Design review of the part built by this model. Coordinates are the model's own, in mm. A direction names the side the tool comes from. Give positions to 0.01 mm unless a question says otherwise; leave off trailing zeros. Loops run counter-clockwise (first coordinate to the right, second up) from the corner with the lowest first, then second, coordinate; pieces in that order, holes last. Notation, with made-up numbers: (72.25, 57.25) - (94.25, 57.25) arc R12 cw to (94.25, 67.25) - close; hole circle Ø6 at (-27, -7.75). An arc over 180 degrees is marked (long way). Write each question's results on one line, items separated by ' | '.
Autodesk Inventor part; units mm, degrees
ref_plane "Work Plane1" through (0, -13.8, 0) normal (1, 0, 0) x (0, 0, 1)
ref_plane "YZ Plane" through (0, 0, 0) normal (1, 0, 0) x (0, 1, 0)
ref_plane "XZ Plane" through (0, 0, 0) normal (0, 1, 0) x (-1, 0, 0)
sketch "Sketch1" plane through (0, 0, 0) normal (0, 0, 1) x (1, 0, 0)
  arc A0 (9.4421, -21.6827) -> (-9.4421, -21.6827) centre (0, -13.8) ccw
  line L0 (0, 15.1128) -> (0, -73.1766)
  line L1 (-45.5, 0) -> (45.5, 0)
  line L2 (-4.9645, 1.7) -> (1.5024, 1.7) construction
  arc A1 (4.998, -26.8243) -> (-4.998, -26.8243) centre (0, -13) ccw
  line L3 (0, -1.5) -> (-5.3069, -1.5) construction
  line L4 (0, -13) -> (-6.8324, -26.0157) construction
  line L5 (-6.8324, -26.0157) -> (-20.0146, -19.0959) construction
  line L6 (-5.6007, -23.6693) -> (-15.85, -18.2891) construction
  circle A2 centre (-5.6007, -23.6693) radius 1
  arc A3 (-3.8298, -24.5989) -> (-6.7537, -22.0352) centre (-5.6007, -23.6693) ccw
  arc A4 (-9.4421, -21.6827) -> (-6.7537, -22.0352) centre (-7.9068, -20.401) ccw
  line L7 (-3.8298, -24.5989) -> (-4.998, -26.8243)
  circle A5 centre (5.6007, -23.6693) radius 1
  arc A6 (6.7537, -22.0352) -> (3.8298, -24.5989) centre (5.6007, -23.6693) ccw
  arc A7 (6.7537, -22.0352) -> (9.4421, -21.6827) centre (7.9068, -20.401) ccw
  line L8 (3.8298, -24.5989) -> (4.998, -26.8243)
  point P0 (-12.9705, -19.8007)
  point P1 (6.8324, -26.0157)
  dimension "d8" = 0.8
  dimension "d38" = 3.2
  dimension "d39" = 13
  dimension "d43" = 14.7
  dimension "d45" = 2.65
  dimension "d46" = 2
  dimension "d47" = 4.998
  dimension "d48" = 2
  dimension "d49" = 2
extrude "Body" add sketch "Sketch1" along normal blind 1.5
ref_plane "Work Plane1" through (0, -13.8, 0) normal (1, 0, 0) x (0, 0, 1)
equation "\"d8\" = 0.25 * SRB1"
equation "\"d38\" = SRB1"
equation "\"d39\" = 0.5 * WD"
equation "\"d43\" = 0.5 * ND"
equation "\"d45\" = 0.5 * SRB2"
equation "\"d46\" = SD5"
equation "\"d47\" = 0.17 * ND"
equation "\"d48\" = SD5"
equation "\"d49\" = SD5"
equation "\"d2\" = SD"
equation "\"WD\" = WDMIN"
equation "\"SD\" = 1.5"
equation "\"SRB1\" = 3.2"
equation "\"ND\" = 29.4"
equation "\"SRB2\" = 5.3"
equation "\"SD5\" = 2"
equation "\"WDMIN\" = 26"
equation "\"SD6\" = 30.1"
equation "\"NND\" = 28"
equation "\"WDMAX\" = NND"
properties part number "DIN 472 - 28 x 1.5" material "Steel, Mild"
(1) Take a section at D-D on x = 0. Give the boundary of the cut face in (y, z), plus the area to 3 significant figures.
Answers below:
outline: (-1.5, 0) - (1.7, 0) - (1.7, 1.5) - (-1.5, 1.5) - close | area: 4.80 mm2
(2) Take a section at B-B on z = 0.25. Give the boundary of the cut face in (x, y), plus the area to 3 significant figures.
Answers below:
outline: (-9.44, -21.68) arc R12.3 cw (long way) to (9.44, -21.68) arc R2 cw to (6.75, -22.04) arc R2 ccw to (3.83, -24.6) - (5, -26.82) arc R14.7 ccw (long way) to (-5, -26.82) - (-3.83, -24.6) arc R2 ccw to (-6.75, -22.04) arc R2 cw to start; hole circle Ø2 at (-5.6, -23.67); hole circle Ø2 at (5.6, -23.67) | area: 204 mm2
(3) Wall thickness on line 1 along X through (y, z) = (-12.75, 1.1); line 2 along Y through (x, z) = (7.25, 1.4); line 3 along X through (y, z) = (-16.75, 0.8): over which ranges is each line inside the solid? List them lowest first. Write a range as from..to.
Answers below:
line 1: -14.7..-12.26, 12.26..14.7 | line 2: -25.79..-22.29, -3.86..-0.21 | line 3: -14.21..-11.94, 11.94..14.21
(4) Take a section at C-C on y = -13. Give the boundary of the cut face in (x, z).
Answers below:
outline: (-14.7, 0) - (-12.27, 0) - (-12.27, 1.5) - (-14.7, 1.5) - close; (12.27, 0) - (14.7, 0) - (14.7, 1.5) - (12.27, 1.5) - close
(5) Draft analysis for pull direction Y (two halves, no side actions). For faces 1 (the cylindrical face through (-4.31, -22.14, 0.74)), 2 (the flat face through (-1, -1, 0)), 3 (the flat face through (-4.41, -25.7, 0.74)), state which applies: pulls with the +Y half, pulls with the -Y half, needs draft (parallel to the pull), parting line crosses it, or undercut.
Answers below:
face 1: undercut | face 2: needs draft | face 3: pulls with the -Y half
(6) Take a section at A-A on x = 7.5. Give the boundary of the cut face in (y, z), plus the area to 3 significant figures.
Answers below:
outline: (-25.64, 0) - (-22.36, 0) - (-22.36, 1.5) - (-25.64, 1.5) - close; (-4.05, 0) - (-0.36, 0) - (-0.36, 1.5) - (-4.05, 1.5) - close | area: 10.5 mm2
(7) Tool access review of faces 4 (the flat face through (4.41, -25.7, 0.74)), 5 (the flat face through (-1, -1, 1.5)), 6 (the cylindrical face through (-8.146, -22.387, 0.74)): name each direction out of +Z, -Z, +X, -X, +Y, -Y from which nothing blocks a thin tool from reaching the whole face with its end or side.
Answers below:
face 4: +Z, -Z, -Y | face 5: +Z, +X, -X, +Y, -Y | face 6: +Z, -Z
